```python
from build123d import *

# Parameters (mm, degrees)
SKETCH1_R           = 7
BOSS_EXTRUDE1_DEPTH = 100
BOSS_EXTRUDE2_DEPTH = 20
BOSS_EXTRUDE3_DEPTH = 20


with BuildPart() as part:
    # Sketch1 → Boss-Extrude1 (new body)
    with BuildSketch(Plane.XY):
        Circle(SKETCH1_R)
    extrude(amount=-BOSS_EXTRUDE1_DEPTH)

    # Sketch2 → Boss-Extrude2 (add)
    with BuildSketch(Plane.XY):
        Polygon((0, 5), (-4.330127019, 2.5), (-4.330127019, -2.5), (0, -5), (4.330127019, -2.5), (4.330127019, 2.5), align=None)
    extrude(amount=BOSS_EXTRUDE2_DEPTH)

    # Sketch3 → Boss-Extrude3 (add)
    with BuildSketch(Plane(origin=(0, 0, -100), x_dir=(-1, 0, 0), z_dir=(0, 0, -1))):
        Polygon((0, 5), (-4.330127019, 2.5), (-4.330127019, -2.5), (0, -5), (4.330127019, -2.5), (4.330127019, 2.5), align=None)
    extrude(amount=BOSS_EXTRUDE3_DEPTH)


solid = part.part
```
Could you check a few things on this model? Use its own coordinates, in mm. A direction names the side the tool comes from. Coordinates: 2 decimals unless noted, no trailing zeros. Write each loop counter-clockwise with the first axis right and the second up, starting at its lowest first coordinate (ties: lowest second). Pieces come first, ordered by that corner, then holes. Notation, with made-up numbers: M 67.25,-1 L 101.25,-1 A22 ccw 101.25,21 Z; hole C 62,82 d5. An arc over 180 degrees is marked long. Answer as CSV lines item,"result". Start each with the question number.
1) I want a section at C-C, the plane x = -1.25. Please give me the cut outline in (y, z), and give its area (3 significant figures).
2) I want a section at D-D, the plane z = -40.5. Please give me the cut outline in (x, y).
3) I want a section at B-B, the plane z = -110. Please give me the cut outline in (x, y).
4) Please list where these lines run through material, in increasing order: line 1 (Y direction, x = 5.5, z = -49); line 2 (Z direction, x = -4.25, y = -2.75); line 3 (X direction, y = 0.25, z = -40). Write a range as from..to.
5) For P1, Ø5, axis at x = 4.5, z = -65, coming from the -Y side; P2, Ø4, axis at y = 1, z = -105.5, coming from the -X side; P3, Ø6, axis at y = -5, z = -12, coming from the +X side, each with a flat end and sliding along its axis, tell me the tip position at first contact or that it passes through.
6) For faces 1 (the flat face through (2.2, 3.73, 9.86)), 2 (the flat face through (-2.2, -3.73, 9.86)), 3 (the flat face through (-4.33, 0, -110)), which set-ups out of +Z, -Z, +X, -X, +Y, -Y let a thin tool reach every point of the face, with its end or its side?
7) I want a section at A-A, the plane y = 0. Please give me the cut outline in (x, z), and give its area (3 significant figures).
Data:
1,outline,"M -6.89,-100 L -4.28,-100 L -4.28,-120 L 4.28,-120 L 4.28,-100 L 6.89,-100 L 6.89,0 L 4.28,0 L 4.28,20 L -4.28,20 L -4.28,0 L -6.89,0 Z"
1,area,"1,720 mm^2"
2,outline,"C 0,0 d14"
3,outline,"M -4.33,-2.5 L 0,-5 L 4.33,-2.5 L 4.33,2.5 L 0,5 L -4.33,2.5 Z"
4,line 1,"y = -4.33..4.33"
4,line 2,"z = -100..0"
4,line 3,"x = -7..7"
5,P1,"stops at y = -6.71"
5,P2,"stops at x = -4.33"
5,P3,"stops at x = 6.71"
6,face 1,"+Z, +X, +Y"
6,face 2,"+Z, -X, -Y"
6,face 3,"-Z, -X, +Y, -Y"
7,outline,"M -7,-100 L -4.33,-100 L -4.33,-120 L 4.33,-120 L 4.33,-100 L 7,-100 L 7,0 L 4.33,0 L 4.33,20 L -4.33,20 L -4.33,0 L -7,0 Z"
7,area,"1,750 mm^2"
